from build123d import *

# Parameters (mm, degrees)
SKETCH2_W           = 63.5
SKETCH2_H           = 158.877
SKETCH2_R           = 2.413
SKETCH2_R_2         = 3.175
BOSS_EXTRUDE1_DEPTH = 6.35
SKETCH3_W           = 1.27
SKETCH3_H           = 6.477
CUT_EXTRUDE1_DEPTH  = 7.35


with BuildPart() as part:
    # Sketch2 → Boss-Extrude1 (new body)
    with BuildSketch(Plane.XY):
        with Locations((31.75, 79.4385)):
            Rectangle(SKETCH2_W, SKETCH2_H)
        with Locations((8.382, 131.445)):
            Circle(SKETCH2_R, mode=Mode.SUBTRACT)
        with Locations((55.118, 131.445)):
            Circle(SKETCH2_R, mode=Mode.SUBTRACT)
        with Locations((55.118, 84.709)):
            Circle(SKETCH2_R, mode=Mode.SUBTRACT)
        with Locations((8.382, 84.709)):
            Circle(SKETCH2_R, mode=Mode.SUBTRACT)
        with Locations((31.75, 108.077)):
            Circle(SKETCH2_R_2, mode=Mode.SUBTRACT)
    extrude(amount=BOSS_EXTRUDE1_DEPTH)

    # Sketch3 → Cut-Extrude1 (cut, through all)
    with BuildSketch(Plane.XY.offset(6.35)):
        with Locations((0.635, 3.2385)):
            Rectangle(SKETCH3_W, SKETCH3_H)
        with Locations((62.865, 3.2385)):
            Rectangle(SKETCH3_W, SKETCH3_H)
    extrude(amount=-CUT_EXTRUDE1_DEPTH, mode=Mode.SUBTRACT)


solid = part.part
Here's how the part is built. I have some questions about the finished solid (model axes, mm). A direction names the side the tool comes from. Coordinates: 2 decimals unless noted, no trailing zeros. Order: outer loops, then holes, each group sorted by start corner. A loop starts at its lowest first (then second) coordinate and runs counter-clockwise, first axis right, second up.
Item 1: For P1, Ø3, axis at y = 3.5, z = 4.5, coming from the -X side; P2, Ø3, axis at y = 2, z = 1.5, coming from the +X side, each with a flat end and sliding along its axis, tell me the tip position at first contact or that it passes through.
Result sheet:
P1: stops at x = 1.27
P2: stops at x = 62.23
Item 2: If we section it at A-A on x = 31.75: List the corners of the cut face in (y, z) for me, plus the area to 3 significant figures.
Result sheet:
outline: (0, 0) - (104.9, 0) - (104.9, 6.35) - (0, 6.35) - close; (111.25, 0) - (158.88, 0) - (158.88, 6.35) - (111.25, 6.35) - close
area: 969 mm2
Item 3: If we mould it in two halves opening along Y, with no side actions, what happens to faces 4 (the face through (0, 82, 3)), 5 (the face through (31, 158.877, 3)), 6 (the face through (7.86, 129.09, 3.13))? For each: +Y half, -Y half, draft (parallel to the pull), parting line (faces both ways), or undercut.
Result sheet:
face 4: draft
face 5: +Y half
face 6: undercut
Item 4: I need wall thicknesses on line 1 (Y direction, x = 31.75, z = 2); line 2 (Y direction, x = 54, z = 4.75); line 3 (Y direction, x = 56, z = 4.5). Which ranges of each line are inside material? Lowest first, please.
Result sheet:
line 1: y = 0 to 104.9, 111.25 to 158.88
line 2: y = 0 to 82.57, 86.85 to 129.31, 133.58 to 158.88
line 3: y = 0 to 82.46, 86.96 to 129.2, 133.69 to 158.88
Item 5: For faces 1 (the face through (31, 0, 3)), 2 (the face through (1.27, 3, 3)), 3 (the face through (62.23, 3, 3)), which set-ups out of +Z, -Z, +X, -X, +Y, -Y let a thin tool reach every point of the face, with its end or its side?
Result sheet:
face 1: +Z, -Z, +X, -X, -Y
face 2: +Z, -Z, -X, -Y
face 3: +Z, -Z, +X, -Y
